Source: CAD feature listing. Evaluate the final solid. Frame: model axes, mm. Give positions to 0.01 mm unless a question says otherwise; leave off trailing zeros. Order: outer loops, then holes, each group sorted by start corner. A loop starts at its lowest first (then second) coordinate and runs counter-clockwise, first axis right, second up. Notation, with made-up numbers: M 42,-21.5 L 72,-21.5 A9 ccw 72,-6.5 Z; hole C 40,80.25 d5. An arc over 180 degrees is marked long. Return JSON: item names as keys, results as strings.
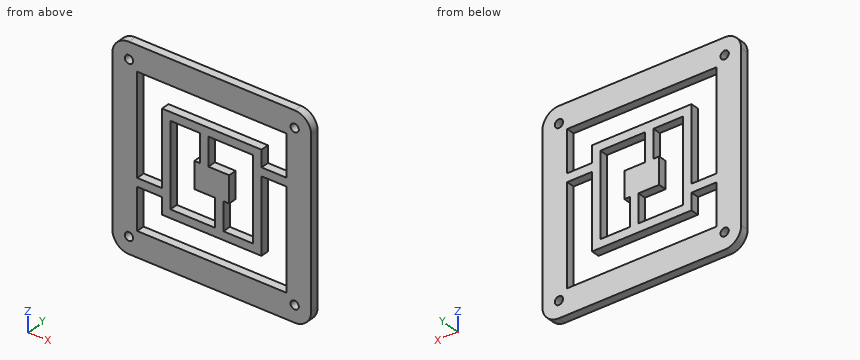
from build123d import *

# Parameters (mm, degrees)
SKETCH1_R             = 2.5
SKETCH1_W             = 90
SKETCH1_H             = 90
BOSS_EXTRUDE1_DEPTH   = 5
SKETCH1_W_2           = 60
SKETCH1_H_2           = 60
SKETCH1_W_3           = 50
SKETCH1_H_3           = 50
BOSS_EXTRUDE1_2_DEPTH = 5
SKETCH1_W_4           = 21
SKETCH1_H_4           = 16
BOSS_EXTRUDE1_3_DEPTH = 5
SKETCH2_W             = 5
SKETCH2_H             = 17
SKETCH2_W_2           = 15
SKETCH2_H_2           = 5
BOSS_EXTRUDE2_DEPTH   = 5


with BuildPart() as part:
    # Sketch1 → Boss-Extrude1 (new body)
    with BuildSketch(Plane(origin=(0, 0, 0), x_dir=(1, 0, 0), z_dir=(0, 1, 0))):
        with BuildLine():
            ThreePointArc((-60, 50), (-57.071067812, 57.071067812), (-50, 60))
            Line((-50, 60), (50, 60))
            ThreePointArc((50, 60), (57.071067812, 57.071067812), (60, 50))
            Line((60, 50), (60, -50))
            ThreePointArc((60, -50), (57.071067812, -57.071067812), (50, -60))
            Line((50, -60), (-50, -60))
            ThreePointArc((-50, -60), (-57.071067812, -57.071067812), (-60, -50))
            Line((-60, -50), (-60, 50))
        make_face()
        with Locations(Location((-50, -50, 0), (0, 0, 270))):
            Circle(SKETCH1_R, mode=Mode.SUBTRACT)
        with Locations(Location((50, -50, 0), (0, 0, 270))):
            Circle(SKETCH1_R, mode=Mode.SUBTRACT)
        with Locations(Location((50, 50, 0), (0, 0, 270))):
            Circle(SKETCH1_R, mode=Mode.SUBTRACT)
        with Locations(Location((-50, 50, 0), (0, 0, 270))):
            Circle(SKETCH1_R, mode=Mode.SUBTRACT)
        Rectangle(SKETCH1_W, SKETCH1_H, mode=Mode.SUBTRACT)
    extrude(amount=BOSS_EXTRUDE1_DEPTH)



with BuildPart() as body_2:
    # Sketch1 → Boss-Extrude1 2 (new body)
    with BuildSketch(Plane(origin=(0, 0, 0), x_dir=(1, 0, 0), z_dir=(0, 1, 0))):
        Rectangle(SKETCH1_W_2, SKETCH1_H_2)
        Rectangle(SKETCH1_W_3, SKETCH1_H_3, mode=Mode.SUBTRACT)
    extrude(amount=BOSS_EXTRUDE1_2_DEPTH)


with BuildPart() as body_3:
    # Sketch1 → Boss-Extrude1 3 (new body)
    with BuildSketch(Plane(origin=(0, 0, 0), x_dir=(1, 0, 0), z_dir=(0, 1, 0))):
        Rectangle(SKETCH1_W_4, SKETCH1_H_4)
    extrude(amount=BOSS_EXTRUDE1_3_DEPTH)


with BuildPart() as part_1:
    add(part.part)

    add(body_2.part)  # Boss-Extrude2 merges body 2

    add(body_3.part)  # Boss-Extrude2 merges body 3
    # Sketch2 → Boss-Extrude2 (add)
    with BuildSketch(Plane(origin=(0, 0, 0), x_dir=(1, 0, 0), z_dir=(0, 1, 0))):
        with Locations((-4.5, -16.5)):
            Rectangle(SKETCH2_W, SKETCH2_H)
        with Locations((4.5, 16.5)):
            Rectangle(SKETCH2_W, SKETCH2_H)
        with Locations((-37.5, 17.5)):
            Rectangle(SKETCH2_W_2, SKETCH2_H_2)
        with Locations((37.5, -17.5)):
            Rectangle(SKETCH2_W_2, SKETCH2_H_2)
    extrude(amount=BOSS_EXTRUDE2_DEPTH)


solid = part_1.part
1. Section query A-A (z = -23.5). Return loops of the section in (x, y), then the cut area to 3 significant figures.
Evaluation:
{"outline": "M -60,0 L -45,0 L -45,5 L -60,5 Z; M -30,0 L -25,0 L -25,5 L -30,5 Z; M 2,0 L 7,0 L 7,5 L 2,5 Z; M 25,0 L 30,0 L 30,5 L 25,5 Z; M 45,0 L 60,0 L 60,5 L 45,5 Z", "area": "225 mm^2"}
2. Ray query, probe 1 along Z at (x, y) = (-23, 4.55); probe 2 along Z at (x, y) = (9, 2.5); probe 3 along Z at (x, y) = (-40, 0.8). Return the intervals inside material, ascending.
Evaluation:
{"probe 1": "z = -60 to -45, -30 to -25, 25 to 30, 45 to 60", "probe 2": "z = -60 to -45, -30 to -25, -8 to 8, 25 to 30, 45 to 60", "probe 3": "z = -60 to -45, -20 to -15, 45 to 60"}
3. Section query D-D (y = 3.35). State how many separate pieces and enclosed holes the cut face has, then the cut area to 3 significant figures.
Evaluation:
{"separate pieces": "1", "enclosed holes": "8", "area": "7,890 mm^2"}
4. Section query C-C (z = -40). Return loops of the section in (x, y).
Evaluation:
{"outline": "M -60,0 L -45,0 L -45,5 L -60,5 Z; M 45,0 L 60,0 L 60,5 L 45,5 Z"}
5. Section query B-B (x = 40.5). Return loops of the section in (y, z).
Evaluation:
{"outline": "M 0,-60 L 5,-60 L 5,-45 L 0,-45 Z; M 0,15 L 5,15 L 5,20 L 0,20 Z; M 0,45 L 5,45 L 5,60 L 0,60 Z"}
